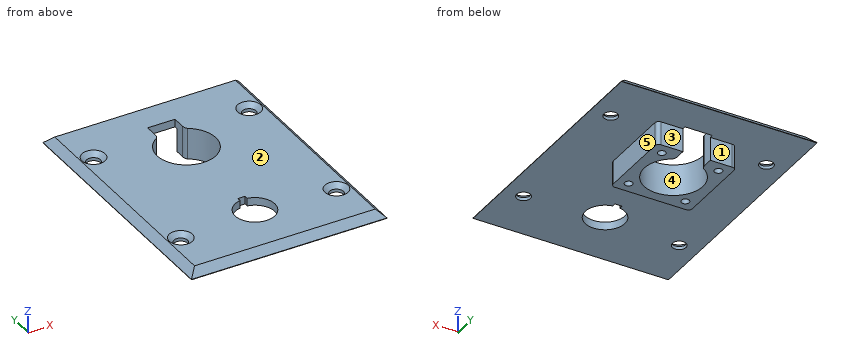
```python
from build123d import *

# Parameters (mm, degrees)
SKETCH_W        = 50
SKETCH_H        = 65
PAD_DEPTH       = 2
SKETCH003_R     = 1
PAD001_DEPTH    = 6
POCKET001_DEPTH = 8.001
SKETCH001_R     = 1.75
POCKET_DEPTH    = 2
CHAMFER_SIZE    = 1.2
CHAMFER001_SIZE = 1.9


with BuildPart() as part:
    # Sketch → Pad (new body)
    with BuildSketch(Plane.XY):
        Rectangle(SKETCH_W, SKETCH_H)
    extrude(amount=PAD_DEPTH)

    # Sketch003 (on DatumPlane) → Pad001 (join)
    with BuildSketch(Plane.XY):
        with BuildLine():
            Line((-10.1, 3.4), (-10.1, 21.6))
            ThreePointArc((-9.1, 22.6), (-9.807107, 22.307107), (-10.1, 21.6))
            Line((-9.1, 22.6), (9.1, 22.6))
            ThreePointArc((10.1, 21.6), (9.807107, 22.307107), (9.1, 22.6))
            Line((10.1, 21.6), (10.1, 3.4))
            ThreePointArc((9.1, 2.4), (9.807107, 2.692893), (10.1, 3.4))
            Line((-9.1, 2.4), (9.1, 2.4))
            ThreePointArc((-10.1, 3.4), (-9.807107, 2.692893), (-9.1, 2.4))
        make_face()
        with Locations((-7.25, 5.25)):
            Circle(SKETCH003_R, mode=Mode.SUBTRACT)
        with Locations((7.25, 5.25)):
            Circle(SKETCH003_R, mode=Mode.SUBTRACT)
        with Locations((7.25, 19.75)):
            Circle(SKETCH003_R, mode=Mode.SUBTRACT)
        with Locations((-7.25, 19.75)):
            Circle(SKETCH003_R, mode=Mode.SUBTRACT)
    extrude(amount=-PAD001_DEPTH)

    # Sketch002 (on DatumPlane) → Pocket001 (cut, through all)
    with BuildSketch(Plane.XY.offset(2)):
        with BuildLine():
            ThreePointArc((-4, 18.844289), (0, 5), (4, 18.844289))
            ThreePointArc((3.5, 20.13325), (3.635081, 19.444191), (4, 18.844289))
            Line((3.5, 23.5), (3.5, 20.13325))
            Line((-3.5, 23.5), (3.5, 23.5))
            Line((-3.5, 23.5), (-3.5, 20.13325))
            ThreePointArc((-4, 18.844289), (-3.635081, 19.444191), (-3.5, 20.13325))
        make_face()
        with BuildLine():
            ThreePointArc((-0.9, -12.530845), (0, -22.55), (0.9, -12.530845))
            Line((0.9, -11.6), (0.9, -12.530845))
            Line((-0.9, -11.6), (0.9, -11.6))
            Line((-0.9, -11.6), (-0.9, -12.530845))
        make_face()
    extrude(amount=-POCKET001_DEPTH, mode=Mode.SUBTRACT)

    # Sketch001 (on DatumPlane) → Pocket (cut)
    with BuildSketch(Plane.XY.offset(2)):
        with Locations((-19.9, 19.1)):
            Circle(SKETCH001_R)
        with Locations((19.9, 19.1)):
            Circle(SKETCH001_R)
        with Locations((19.9, -19.1)):
            Circle(SKETCH001_R)
        with Locations((-19.9, -19.1)):
            Circle(SKETCH001_R)
    extrude(amount=-POCKET_DEPTH, mode=Mode.SUBTRACT)

    # Chamfer
    chamfer_edges = [part.edges().sort_by_distance(p)[0] for p in [
        (-21.65, 19.1, 2),
        (18.15, 19.1, 2),
        (18.15, -19.1, 2),
        (-21.65, -19.1, 2),
    ]]
    chamfer(chamfer_edges, length=CHAMFER_SIZE)

    # Chamfer001
    chamfer001_edges = [part.edges().sort_by_distance(p)[0] for p in [
        (-25, 0, 2),
        (0, 32.5, 2),
        (25, 0, 2),
        (0, -32.5, 2),
    ]]
    chamfer(chamfer001_edges, length=CHAMFER001_SIZE)


solid = part.part
```
Part model, mm, in its own coordinate system. Face numbers are marked on the shaded views. A direction names the side the tool comes from. Round coordinates to 2 decimals unless told otherwise and drop trailing zeros. Loops run counter-clockwise (first coordinate to the right, second up) from the corner with the lowest first, then second, coordinate; pieces in that order, holes last. Notation, with made-up numbers: (35.5, -8.5) -> (92.5, -8.5) arc R16 cw to (92.5, -4.5) -> close; hole circle Ø7 at (79.25, -10). An arc over 180 degrees is marked (long way). Use CSV: the item, a comma, the result in double quotes. Start each with the question number.
1) Cut at B-B, the plane y = 12.5. Write the cut outline in (x, z), plus the area to 3 significant figures.
2) Pull direction Y, two halves, no side cores. Call the marked faces 3, 4 and 5: +Y half, -Y half, draft (parallel to the pull), parting line (faces both ways), or undercut.
3) Cut at A-A, the plane x = -19.9. Write the cut outline in (y, z).
4) Wall check: L1, parallel to X at y = 12.5, z = -3.5; L2, parallel to Y at x = -19.9, z = 0.25; L3, parallel to Y at x = -19.9, z = 0.35. Give the ranges that are in metal, low to high. Write a range as [from, to].
5) Drop flat-ended pins along their axis: P1, Ø3.5, axis at y = 21.5, z = -0.5, coming from the -X side; P2, Ø2, axis at x = -19.9, y = 19.1, coming from the -Z side; P3, Ø1.8, axis at y = 14, z = -3.5, coming from the -X side; P4, Ø1.7, axis at x = -6, z = -2, coming from the +Y side. Give the stop position or say it passes through.
6) Which spindle directions (+Z, -Z, +X, -X, +Y, -Y) get a long thin tool onto all of the face, cutting with end or side? Do the marked faces 1 and 2. Say none if no direction does.
7) Cut at C-C, the plane z = -2.5. Write the cut outline in (x, y).
8) Cut at D-D, the plane y = 0. Write the cut outline in (x, z).
Determined:
1,outline,"(-25, 0) -> (-10.1, 0) -> (-10.1, -6) -> (-7.5, -6) -> (-7.5, 2) -> (-23.1, 2) -> (-25, 0.1) -> close; (7.5, -6) -> (10.1, -6) -> (10.1, 0) -> (25, 0) -> (25, 0.1) -> (23.1, 2) -> (7.5, 2) -> close"
1,area,"97.6 mm2"
2,face 3,"+Y half"
2,face 4,"undercut"
2,face 5,"draft"
3,outline,"(-32.5, 0) -> (-20.85, 0) -> (-20.85, 0.8) -> (-22.05, 2) -> (-30.6, 2) -> (-32.5, 0.1) -> close; (-17.35, 0) -> (17.35, 0) -> (17.35, 0.8) -> (16.15, 2) -> (-16.15, 2) -> (-17.35, 0.8) -> close; (20.85, 0) -> (32.5, 0) -> (32.5, 0.1) -> (30.6, 2) -> (22.05, 2) -> (20.85, 0.8) -> close"
4,L1,"x = [-10.1, -7.5], [7.5, 10.1]"
4,L2,"y = [-32.35, -20.85], [-17.35, 17.35], [20.85, 32.35]"
4,L3,"y = [-32.25, -20.85], [-17.35, 17.35], [20.85, 32.25]"
5,P1,"stops at x = -25"
5,P2,"passes through"
5,P3,"stops at x = -10.1"
5,P4,"stops at y = 22.6"
6,face 1,"-Z, +X, -X, +Y"
6,face 2,"+Z, +X, -X, +Y, -Y"
7,outline,"(-10.1, 3.4) arc R1 ccw to (-9.1, 2.4) -> (9.1, 2.4) arc R1 ccw to (10.1, 3.4) -> (10.1, 21.6) arc R1 ccw to (9.1, 22.6) -> (3.5, 22.6) -> (3.5, 20.13) arc R2 ccw to (4, 18.84) arc R7.5 cw (long way) to (-4, 18.84) arc R2 ccw to (-3.5, 20.13) -> (-3.5, 22.6) -> (-9.1, 22.6) arc R1 ccw to (-10.1, 21.6) -> close; hole circle Ø2 at (-7.25, 5.25); hole circle Ø2 at (-7.25, 19.75); hole circle Ø2 at (7.25, 5.25); hole circle Ø2 at (7.25, 19.75)"
8,outline,"(-25, 0) -> (25, 0) -> (25, 0.1) -> (23.1, 2) -> (-23.1, 2) -> (-25, 0.1) -> close"
